Verification items for the finished model (mm, model axes). A direction names the side the tool comes from. Round coordinates to 2 decimals unless told otherwise and drop trailing zeros. Write each loop counter-clockwise with the first axis right and the second up, starting at its lowest first coordinate (ties: lowest second). Pieces come first, ordered by that corner, then holes. Notation, with made-up numbers: (-29.5, -12) - (5.5, -12) arc R19 cw to (5.5, -3) - close; hole circle Ø10 at (6.5, -33). An arc over 180 degrees is marked (long way). Answer as a JSON object with one key per item and string values.
Autodesk Inventor part; units mm, degrees
ref_plane "YZ Plane" through (0, 0, 0) normal (1, 0, 0) x (0, 1, 0)
ref_plane "XZ Plane" through (0, 0, 0) normal (0, 1, 0) x (-1, 0, 0)
ref_plane "XY Plane" through (0, 0, 0) normal (0, 0, 1) x (1, 0, 0)
sketch "Sketch1" plane through (0, 0, 0) normal (0, 1, 0) x (-1, 0, 0)
  line L0 (33.8585, -6) -> (-33.8585, -6)
  line L1 (-34.295, -2.5) -> (34.295, -2.5)
  line L2 (0.5017, -38.45) -> (-0.4983, -38.45)
  line L3 (-0.4983, -38.45) -> (-0.4983, -38.85)
  line L4 (-0.4983, -38.85) -> (0.5017, -38.85)
  line L5 (0.5017, -38.85) -> (0.5017, -38.45)
  line L6 (0.5017, -38.45) -> (-0.4983, -38.85) construction
  line L7 (-0.4983, -38.45) -> (0.5017, -38.85) construction
  line L8 (9.6888, -37.2126) -> (8.7179, -37.452)
  line L9 (8.7179, -37.452) -> (8.8136, -37.8403)
  line L10 (8.8136, -37.8403) -> (9.7846, -37.601)
  line L11 (9.7846, -37.601) -> (9.6888, -37.2126)
  line L12 (18.3129, -33.8126) -> (17.4274, -34.2773)
  line L13 (17.4274, -34.2773) -> (17.6133, -34.6315)
  line L14 (17.6133, -34.6315) -> (18.4987, -34.1668)
  line L15 (18.4987, -34.1668) -> (18.3129, -33.8126)
  line L16 (25.8726, -28.4475) -> (25.1241, -29.1107)
  line L17 (25.1241, -29.1107) -> (25.3893, -29.4101)
  line L18 (25.3893, -29.4101) -> (26.1379, -28.7469)
  line L19 (26.1379, -28.7469) -> (25.8726, -28.4475)
  line L20 (31.9287, -21.4292) -> (31.3607, -22.2522)
  line L21 (31.3607, -22.2522) -> (31.6899, -22.4794)
  line L22 (31.6899, -22.4794) -> (32.2579, -21.6564)
  line L23 (32.2579, -21.6564) -> (31.9287, -21.4292)
  line L24 (36.1293, -13.1654) -> (35.7747, -14.1005)
  line L25 (35.7747, -14.1005) -> (36.1487, -14.2423)
  line L26 (36.1487, -14.2423) -> (36.5033, -13.3073)
  line L27 (36.5033, -13.3073) -> (36.1293, -13.1654)
  line L28 (38.2301, -4.1366) -> (38.1096, -5.1293)
  line L29 (38.1096, -5.1293) -> (38.5067, -5.1775)
  line L30 (38.5067, -5.1775) -> (38.6272, -4.1848)
  line L31 (38.6272, -4.1848) -> (38.2301, -4.1366)
  line L32 (38.1092, 5.1327) -> (38.2297, 4.14)
  line L33 (38.2297, 4.14) -> (38.6268, 4.1882)
  line L34 (38.6268, 4.1882) -> (38.5063, 5.1809)
  line L35 (38.5063, 5.1809) -> (38.1092, 5.1327)
  line L36 (35.7735, 14.1037) -> (36.1281, 13.1687)
  line L37 (36.1281, 13.1687) -> (36.5021, 13.3105)
  line L38 (36.5021, 13.3105) -> (36.1475, 14.2455)
  line L39 (36.1475, 14.2455) -> (35.7735, 14.1037)
  line L40 (31.3587, 22.255) -> (31.9268, 21.432)
  line L41 (31.9268, 21.432) -> (32.256, 21.6592)
  line L42 (32.256, 21.6592) -> (31.6879, 22.4822)
  line L43 (31.6879, 22.4822) -> (31.3587, 22.255)
  line L44 (25.1215, 29.1129) -> (25.87, 28.4498)
  line L45 (25.87, 28.4498) -> (26.1353, 28.7492)
  line L46 (26.1353, 28.7492) -> (25.3868, 29.4123)
  line L47 (25.3868, 29.4123) -> (25.1215, 29.1129)
  line L48 (17.4244, 34.2789) -> (18.3098, 33.8142)
  line L49 (18.3098, 33.8142) -> (18.4957, 34.1684)
  line L50 (18.4957, 34.1684) -> (17.6102, 34.6331)
  line L51 (17.6102, 34.6331) -> (17.4244, 34.2789)
  line L52 (8.7145, 37.4528) -> (9.6855, 37.2135)
  line L53 (9.6855, 37.2135) -> (9.7812, 37.6018)
  line L54 (9.7812, 37.6018) -> (8.8103, 37.8412)
  line L55 (8.8103, 37.8412) -> (8.7145, 37.4528)
  line L56 (-0.5017, 38.45) -> (0.4983, 38.45)
  line L57 (0.4983, 38.45) -> (0.4983, 38.85)
  line L58 (0.4983, 38.85) -> (-0.5017, 38.85)
  line L59 (-0.5017, 38.85) -> (-0.5017, 38.45)
  line L60 (-9.6888, 37.2126) -> (-8.7179, 37.452)
  line L61 (-8.7179, 37.452) -> (-8.8136, 37.8403)
  line L62 (-8.8136, 37.8403) -> (-9.7846, 37.601)
  line L63 (-9.7846, 37.601) -> (-9.6888, 37.2126)
  line L64 (-18.3129, 33.8126) -> (-17.4274, 34.2773)
  line L65 (-17.4274, 34.2773) -> (-17.6133, 34.6315)
  line L66 (-17.6133, 34.6315) -> (-18.4987, 34.1668)
  line L67 (-18.4987, 34.1668) -> (-18.3129, 33.8126)
  line L68 (-25.8726, 28.4475) -> (-25.1241, 29.1107)
  line L69 (-25.1241, 29.1107) -> (-25.3893, 29.4101)
  line L70 (-25.3893, 29.4101) -> (-26.1379, 28.7469)
  line L71 (-26.1379, 28.7469) -> (-25.8726, 28.4475)
  line L72 (-31.9287, 21.4292) -> (-31.3607, 22.2522)
  line L73 (-31.3607, 22.2522) -> (-31.6899, 22.4794)
  line L74 (-31.6899, 22.4794) -> (-32.2579, 21.6564)
  line L75 (-32.2579, 21.6564) -> (-31.9287, 21.4292)
  line L76 (-36.1293, 13.1654) -> (-35.7747, 14.1005)
  line L77 (-35.7747, 14.1005) -> (-36.1487, 14.2423)
  line L78 (-36.1487, 14.2423) -> (-36.5033, 13.3073)
  line L79 (-36.5033, 13.3073) -> (-36.1293, 13.1654)
  line L80 (-38.2301, 4.1366) -> (-38.1096, 5.1293)
  line L81 (-38.1096, 5.1293) -> (-38.5067, 5.1775)
  line L82 (-38.5067, 5.1775) -> (-38.6272, 4.1848)
  line L83 (-38.6272, 4.1848) -> (-38.2301, 4.1366)
  line L84 (-38.1092, -5.1327) -> (-38.2297, -4.14)
  line L85 (-38.2297, -4.14) -> (-38.6268, -4.1882)
  line L86 (-38.6268, -4.1882) -> (-38.5063, -5.1809)
  line L87 (-38.5063, -5.1809) -> (-38.1092, -5.1327)
  line L88 (-35.7735, -14.1037) -> (-36.1281, -13.1687)
  line L89 (-36.1281, -13.1687) -> (-36.5021, -13.3105)
  line L90 (-36.5021, -13.3105) -> (-36.1475, -14.2455)
  line L91 (-36.1475, -14.2455) -> (-35.7735, -14.1037)
  line L92 (-31.3587, -22.255) -> (-31.9268, -21.432)
  line L93 (-31.9268, -21.432) -> (-32.256, -21.6592)
  line L94 (-32.256, -21.6592) -> (-31.6879, -22.4822)
  line L95 (-31.6879, -22.4822) -> (-31.3587, -22.255)
  line L96 (-25.1215, -29.1129) -> (-25.87, -28.4498)
  line L97 (-25.87, -28.4498) -> (-26.1353, -28.7492)
  line L98 (-26.1353, -28.7492) -> (-25.3868, -29.4123)
  line L99 (-25.3868, -29.4123) -> (-25.1215, -29.1129)
  line L100 (-17.4244, -34.2789) -> (-18.3098, -33.8142)
  line L101 (-18.3098, -33.8142) -> (-18.4957, -34.1684)
  line L102 (-18.4957, -34.1684) -> (-17.6102, -34.6331)
  line L103 (-17.6102, -34.6331) -> (-17.4244, -34.2789)
  line L104 (-8.7145, -37.4528) -> (-9.6855, -37.2135)
  line L105 (-9.6855, -37.2135) -> (-9.7812, -37.6018)
  line L106 (-9.7812, -37.6018) -> (-8.8103, -37.8412)
  line L107 (-8.8103, -37.8412) -> (-8.7145, -37.4528)
  arc A0 (-33.6574, 19) -> (32.0907, -21.5409) centre (0, 0) ccw
  arc A1 (33.6574, -19) -> (33.6574, 19) centre (0, 0) ccw
  arc A2 (32.0887, 21.5438) -> (-32.0907, 21.5409) centre (0, 0) ccw
  line L108 (36.1642, -3.8857) -> (36.1642, -3.8892)
  line L109 (36.1642, -4.8931) -> (36.1642, -4.8965)
  line L110 (-34.9312, -4.7468) -> (-34.9312, -4.7433)
  line L111 (-34.9312, -3.7395) -> (-34.9312, -3.736)
  line L112 (33.6574, -19) -> (28.66, -19)
  line L113 (-28.66, -19) -> (-33.6574, -19)
  line L114 (-33.6574, 19) -> (-28.66, 19)
  line L115 (28.66, 19) -> (33.6574, 19)
  arc A3 (28.66, -19) -> (33.8585, -6) centre (0, 0) ccw
  arc A4 (34.295, -2.5) -> (28.66, 19) centre (0, 0) ccw
  arc A5 (-28.66, 19) -> (-34.295, -2.5) centre (0, 0) ccw
  arc A6 (-33.8585, -6) -> (-28.66, -19) centre (0, 0) ccw
  point P0 (0.0017, -38.65)
  point P1 (35.9587, -14.1702)
  point P2 (36.3132, -13.2352)
  point P3 (38.3049, -5.153)
  point P4 (38.4254, -4.1603)
  point P5 (38.4251, 4.1637)
  point P6 (38.3045, 5.1564)
  point P7 (36.3121, 13.2384)
  point P8 (35.9574, 14.1734)
  point P9 (-35.9587, 14.1702)
  point P10 (-36.3132, 13.2352)
  point P11 (-38.3049, 5.153)
  point P12 (-38.4254, 4.1603)
  point P13 (-38.4251, -4.1637)
  point P14 (-38.3045, -5.1564)
  point P15 (-36.3121, -13.2384)
  point P16 (-35.9574, -14.1734)
  dimension "d2" = 2.5
  dimension "d3" = 3.5
  dimension "d10" = 1
  dimension "d11" = 0.4
  dimension "d14" = 360
  dimension "d18" = 38.65
  dimension "d19" = 4.9974
extrude "Extrusion1" add sketch "Sketch1" along normal blind 10 contours L0 A6 L113 A0 L91 L88 L89 L87 L84 L85 L83 L80 L81 L79 L76 L77 L114 A5 L1 A4 L115 A1 L39 L36 L37 L35 L32 L33 L31 L28 L29 L27 L24 L25 L112 A3 | A1 L27 L26 L25 | L25 L24 L27 A1 | A0 L89 L88 L91 | L91 L90 L89 A0 | A1 L31 L30 L29 | L29 L28 L31 A1 | A0 L85 L84 L87 | L87 L86 L85 A0 | A1 L35 L34 L33 | L33 L32 L35 A1 | A0 L81 L80 L83 | L83 L82 L81 A0 | A1 L39 L38 L37 | L37 L36 L39 A1 | A0 L77 L76 L79 | L79 L78 L77 A0
sketch "Sketch2" plane through (0, 10, 0) normal (0, 1, 0) x (1, 0, 0)
  arc A0 (33.8585, 6) -> (28.66, 19) centre (0, 0) ccw
  line L0 (34.295, 2.5) -> (-34.295, 2.5)
  line L1 (-3.804, 9) -> (7.0469, 9)
  line L2 (33.1873, 9) -> (-33.1873, 9)
  line L3 (-28.66, 19) -> (-33.6574, 19)
  line L4 (-33.6574, -19) -> (-28.66, -19)
  line L5 (-28.66, -19) -> (-36.8951, -19)
  arc A1 (-34.295, 2.5) -> (-28.66, -19) centre (0, 0) ccw
  arc A2 (28.66, -19) -> (34.295, 2.5) centre (0, 0) ccw
  arc A3 (36.8951, -19) -> (36.8951, 19) centre (0, 0) ccw
  arc A4 (-36.8951, 19) -> (-36.8951, -19) centre (0, 0) ccw
  arc A5 (33.1873, 9) -> (28.66, 19) centre (0, 0) ccw
  arc A6 (-28.66, 19) -> (-33.1873, 9) centre (0, 0) ccw
  line L6 (36.8951, 19) -> (28.66, 19)
  line L7 (-28.66, 19) -> (-36.8951, 19)
  line L8 (-31.7819, -19) -> (-28.66, -19)
  line L9 (28.66, -19) -> (36.8951, -19)
  line L10 (-30.5962, 19) -> (-28.66, 19)
  line L11 (28.66, 19) -> (36.8951, 19)
  point P0 (28.66, 19)
  point P1 (7.0469, 9)
  dimension "d24" = 41.5
  dimension "d25" = 6.5
extrude "Extrusion2" add sketch "Sketch2" along normal blind 2
sketch "Sketch3" plane through (-34.295, 0, -2.5) normal (0, 0, 1) x (1, 0, 0)
  line L0 (0, 12) -> (68.59, 12)
  line L1 (0, 0) -> (0, 12)
  point P0 (34.295, 0)
  point P1 (35.121, 5.396)
  dimension "d28" = 6.604
  dimension "d29" = 35.121
hole "Hole1" at (0.826, 5.396, -2.5) direction (0, 0, -1) diameter 2.6416 depth 10.979
properties part number "AQS_Mount_3DPrint"
1. Material ranges on probe 1 along Z at (x, y) = (-14.5, 3.5); probe 2 along Y at (x, z) = (37, -17); probe 3 along X at (y, z) = (6.5, 7.5), recorded low to high. Write a range as from..to.
Completed:
{"probe 1": "z = -6..-2.5", "probe 2": "y = 10..12", "probe 3": "x = -37.92..-33.56, 33.56..37.92"}
2. Cross-section at C-C (x = -1.5). Record the boundary of the cut face in (y, z).
Completed:
{"outline": "(0, -6) - (10, -6) - (10, -9) - (12, -9) - (12, -2.5) - (0, -2.5) - close"}
3. Cross-section at D-D (z = -1). Record the boundary of the cut face in (x, y), plus the area to 3 significant figures.
Completed:
{"outline": "(-41.49, 10) - (-38.64, 10) - (-38.64, 0) - (-34.37, 0) - (-34.37, 12) - (-41.49, 12) - close; (34.37, 0) - (38.64, 0) - (38.64, 10) - (41.49, 10) - (41.49, 12) - (34.37, 12) - close", "area": "114 mm^2"}
4. Mould release check, pull along X, two halves, no side actions. Record for faces 1 (the face through (31, 6, -19)), 2 (the face through (41.5, 11, -0.3)), 3 (the face through (31.89, 5.92, -12.86)), 4 (the face through (-31.357, 10.986, -14.111)): released by +X, released by -X, zero draft, split by the parting line, or undercut.
Completed:
{"face 1": "zero draft", "face 2": "released by +X", "face 3": "undercut", "face 4": "undercut"}
5. Cross-section at A-A (z = -12). Record the boundary of the cut face in (x, y), plus the area to 3 significant figures.
Completed:
{"outline": "(-39.73, 10) - (-36.74, 10) - (-36.74, 0) - (-32.22, 0) - (-32.22, 12) - (-39.73, 12) - close; (32.22, 0) - (36.74, 0) - (36.74, 10) - (39.73, 10) - (39.73, 12) - (32.22, 12) - close", "area": "120 mm^2"}
6. Go/stop test with flat-tipped pins: pin 1 (1 mm diameter, centred on x = -2, y = 10.5, fed in from -Z); pin 2 (1.5 mm diameter, centred on x = -10, y = 6, fed in from +Z); pin 3 (3 mm diameter, centred on x = 2.5, y = 4.5, fed in from -Z). Record where each tip stops, or that it passes through.
Completed:
{"pin 1": "stops at z = -9", "pin 2": "stops at z = -2.5", "pin 3": "stops at z = -6"}
7. Cross-section at B-B (y = 11.25). Record the boundary of the cut face in (x, z) (3 decimals).
Completed:
{"outline": "(-36.895, -19) - (-28.66, -19) arc R34.387 cw to (-33.187, -9) - (33.187, -9) arc R34.385 cw to (28.66, -19) - (36.895, -19) arc R41.5 ccw to (36.895, 19) - (28.66, 19) arc R34.386 cw to (34.295, -2.5) - (-34.295, -2.5) arc R34.386 cw to (-28.66, 19) - (-36.895, 19) arc R41.5 ccw to start"}
8. Access from +Z, -Z, +X, -X, +Y, -Y to the whole of each face (thin tool, end or side, straight path). Record for faces 5 (the face through (38.65, 4.93, -0.06)), 6 (the face through (-39, 10, 0)).
Completed:
{"face 5": "+X, -Y", "face 6": "-X, -Y"}
